```python
from build123d import *

# Parameters (mm, degrees)
SKETCH_1_W          = 104
SKETCH_1_H          = 75
SKETCH_1_W_2        = 14.813912832
SKETCH_1_H_2        = 67
SKETCH_1_W_3        = 62
SKETCH_1_H_3        = 62
SKETCH_1_W_4        = 11.186087168
EXTRUDE_3_DEPTH     = 17
SKETCH_3_W          = 4
SKETCH_3_H          = 17
EXTRUDE_4_DEPTH     = 18
SKETCH_4_R          = 1.5
CUT_EXTRUDE_2_DEPTH = 150


with BuildPart() as part:
    # 草图1 → 凸台-拉伸3 (new body)
    with BuildSketch(Plane(origin=(0, 0, 0), x_dir=(1, 0, 0), z_dir=(0, 1, 0))):
        with Locations((27.017596878, 29.599337879)):
            Rectangle(SKETCH_1_W, SKETCH_1_H)
        with Locations((-13.575446706, 29.599337879)):
            Rectangle(SKETCH_1_W_2, SKETCH_1_H_2, mode=Mode.SUBTRACT)
        with Locations((28.83150971, 29.599337879)):
            Rectangle(SKETCH_1_W_3, SKETCH_1_H_3, mode=Mode.SUBTRACT)
        with Locations((69.424553294, 29.599337879)):
            Rectangle(SKETCH_1_W_4, SKETCH_1_H_2, mode=Mode.SUBTRACT)
    extrude(amount=EXTRUDE_3_DEPTH)

    # 草图3 → 凸台-拉伸4 (add)
    with BuildSketch(Plane(origin=(0, 17, 0), x_dir=(1, 0, 0), z_dir=(0, 1, 0))):
        with Locations((-22.982403122, 0.599337879)):
            Rectangle(SKETCH_3_W, SKETCH_3_H)
        with Locations((77.017596878, 0.599337879)):
            Rectangle(SKETCH_3_W, SKETCH_3_H)
    extrude(amount=EXTRUDE_4_DEPTH)

    # 草图4 → 切除-拉伸2 (cut)
    with BuildSketch(Plane.ZY.offset(24.982403122)):
        with BuildLine():
            Line((-9.099337879, 35), (-9.099337879, 26.5))
            ThreePointArc((-9.099337879, 26.5), (-6.609745519, 32.51040764), (-0.599337879, 35))
            Line((-0.599337879, 35), (-9.099337879, 35))
        make_face()
        with BuildLine():
            Line((7.900662121, 35), (-0.599337879, 35))
            ThreePointArc((-0.599337879, 35), (5.411069761, 32.51040764), (7.900662121, 26.5))
            Line((7.900662121, 26.5), (7.900662121, 35))
        make_face()
        with Locations((-0.599337879, 26.5)):
            Circle(SKETCH_4_R)
    extrude(amount=-CUT_EXTRUDE_2_DEPTH, mode=Mode.SUBTRACT)


solid = part.part
```
Can you work these out from the model? Positions are in its coordinate system, mm. A direction names the side the tool comes from. Give positions to 0.01 mm unless a question says otherwise; leave off trailing zeros. Loops run counter-clockwise (first coordinate to the right, second up) from the corner with the lowest first, then second, coordinate; pieces in that order, holes last. Notation, with made-up numbers: M 47,-32.5 L 82,-32.5 A9 cw 82,-23.5 Z; hole C 70,71 d1. An arc over 180 degrees is marked long. Answer in a Markdown table with one row per item.
1. Suppose I cut it at A-A on z = -27. Write out the boundary of the cut face in (x, y), plus the area to 3 significant figures.
Taken from the geometry:
| item | result |
|---|---|
| outline | M -24.98,0 L -20.98,0 L -20.98,17 L -24.98,17 Z; M -6.17,0 L -2.17,0 L -2.17,17 L -6.17,17 Z; M 59.83,0 L 63.83,0 L 63.83,17 L 59.83,17 Z; M 75.02,0 L 79.02,0 L 79.02,17 L 75.02,17 Z |
| area | 272 mm² |
2. If I drill on line 1 along X through (y, z) = (7.5, -62.5); line 2 along X through (y, z) = (13.5, -30.5); line 3 along X through (y, z) = (21.5, -3), over which ranges is the centre line in solid material (lowest first)?
Taken from the geometry:
| item | result |
|---|---|
| line 1 | x = -24.98 to -20.98, -6.17 to 63.83, 75.02 to 79.02 |
| line 2 | x = -24.98 to -20.98, -6.17 to -2.17, 59.83 to 63.83, 75.02 to 79.02 |
| line 3 | x = -24.98 to -20.98, 75.02 to 79.02 |
3. Suppose I cut it at D-D on y = 9.5. Write out the boundary of the cut face in (x, z).
Taken from the geometry:
| item | result |
|---|---|
| outline | M -24.98,-67.1 L 79.02,-67.1 L 79.02,7.9 L -24.98,7.9 Z; hole M -20.98,-63.1 L -6.17,-63.1 L -6.17,3.9 L -20.98,3.9 Z; hole M -2.17,-60.6 L 59.83,-60.6 L 59.83,1.4 L -2.17,1.4 Z; hole M 63.83,-63.1 L 75.02,-63.1 L 75.02,3.9 L 63.83,3.9 Z |
4. Suppose I cut it at B-B on y = 19.5. Write out the boundary of the cut face in (x, z).
Taken from the geometry:
| item | result |
|---|---|
| outline | M -24.98,-9.1 L -20.98,-9.1 L -20.98,7.9 L -24.98,7.9 Z; M 75.02,-9.1 L 79.02,-9.1 L 79.02,7.9 L 75.02,7.9 Z |
5. Thinking about a two-plate mould opening in X: for faces 1 (the flat face through (-4, 0, -33)), 2 (the flat face through (-24.982, 9, -21)), 3 (the flat face through (63.832, 8, -29)), which applies, released by +X, released by -X, zero draft, split by the parting line, or undercut?
Taken from the geometry:
| item | result |
|---|---|
| face 1 | zero draft |
| face 2 | released by -X |
| face 3 | undercut |
6. For pin 1 Ø1.2 at (x, y) = (-22.5, 21.5) entering from -Z; pin 2 Ø8 at (x, z) = (66, -16) entering from +Y; pin 3 Ø10 at (x, y) = (28, 24) entering from -Z (1 decimal), each with a flat end and sliding along its axis, tell me the tip position at first contact or that it passes through.
Taken from the geometry:
| item | result |
|---|---|
| pin 1 | stops at z = -9.1 |
| pin 2 | stops at y = 17 |
| pin 3 | passes through |
7. Which directions (+Z, -Z, +X, -X, +Y, -Y) give clear straight access to the entire face, cutting with the end or side of a thin tool? Please do faces 4 (the flat face through (79.018, 9, -21)), 5 (the flat face through (23, 17, -63)), 6 (the cylindrical face through (-23.01, 27.987, -0.795)), 7 (the flat face through (-2.168, 8, -29)), 8 (the flat face through (-23, 22, -9.099)).
Taken from the geometry:
| item | result |
|---|---|
| face 4 | +Z, -Z, +X, +Y, -Y |
| face 5 | -Z, +Y |
| face 6 | +X, -X |
| face 7 | +Y, -Y |
| face 8 | -Z, +X, -X, +Y |
8. Suppose I cut it at C-C on x = -11.5. Write out the boundary of the cut face in (y, z), plus the area to 3 significant figures.
Taken from the geometry:
| item | result |
|---|---|
| outline | M 0,-67.1 L 17,-67.1 L 17,-63.1 L 0,-63.1 Z; M 0,3.9 L 17,3.9 L 17,7.9 L 0,7.9 Z |
| area | 136 mm² |
